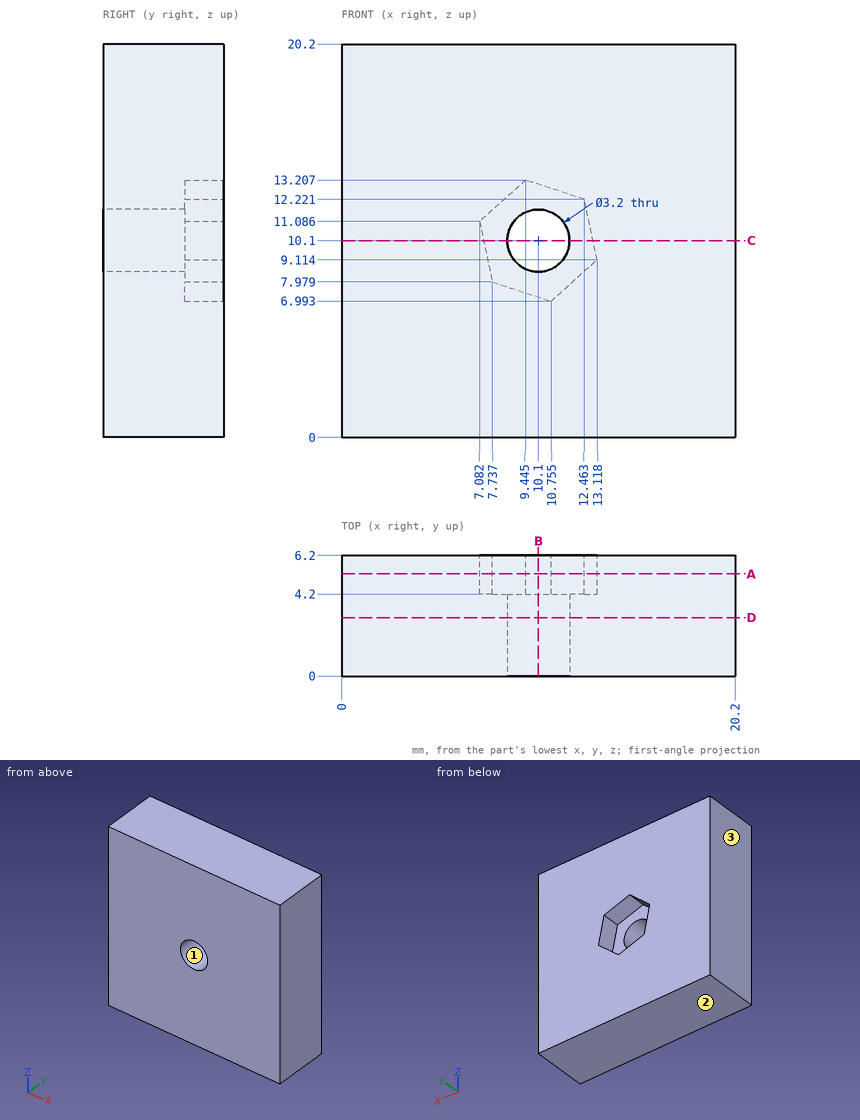
Here's the drawing with two shaded views (mm, measured from the low corner). I have some questions. Coordinates: 2 decimals unless noted, no trailing zeros. Write each loop counter-clockwise with the first axis right and the second up, starting at its lowest first coordinate (ties: lowest second). Pieces come first, ordered by that corner, then holes.
Item 1: I want a section at C-C on z = 10.1. Write out the boundary of the cut face in (x, y).
Item 2: I want a section at B-B on x = 10.1. Write out the boundary of the cut face in (y, z).
Item 3: If I drill on line 1 (Z direction, x = 10.1, y = 2.05); line 2 (Z direction, x = 11.5, y = 4.5) (1 decimal), over which ranges is the centre line in solid material (lowest first)?
Item 4: I want a section at D-D on y = 3. Write out the boundary of the cut face in (x, z), and give its area (3 significant figures).
Item 5: Will this pin go through, and if not, where does the flat tip stop? pin 1 (4 mm diameter, centred on x = 10.1, z = 10.1, fed in from +Y).
Item 6: If we mould it in two halves opening along Z, with no side actions, what happens to the marked faces 1, 2 and 3? For each: +Z half, -Z half, draft (parallel to the pull), parting line (faces both ways), or undercut.
Item 7: I want a section at A-A on y = 5.25. Write out the boundary of the cut face in (x, z) (1 decimal).
Findings below:
1. outline: (0, 0) - (8.5, 0) - (8.5, 4.2) - (7.29, 4.2) - (7.29, 6.2) - (0, 6.2) - close; (11.7, 0) - (20.2, 0) - (20.2, 6.2) - (12.91, 6.2) - (12.91, 4.2) - (11.7, 4.2) - close
2. outline: (0, 0) - (6.2, 0) - (6.2, 7.21) - (4.2, 7.21) - (4.2, 8.5) - (0, 8.5) - close; (0, 11.7) - (4.2, 11.7) - (4.2, 12.99) - (6.2, 12.99) - (6.2, 20.2) - (0, 20.2) - close
3. line 1: z = 0 to 8.5, 11.7 to 20.2
3. line 2: z = 0 to 7.7, 12.5 to 20.2
4. outline: (0, 0) - (20.2, 0) - (20.2, 20.2) - (0, 20.2) - close; hole circle Ø3.2 at (10.1, 10.1)
4. area: 400 mm2
5. pin 1: stops at y = 4.2
6. face 1: undercut
6. face 2: -Z half
6. face 3: draft
7. outline: (0, 0) - (20.2, 0) - (20.2, 20.2) - (0, 20.2) - close; hole (7.1, 11.1) - (7.7, 8) - (10.8, 7) - (13.1, 9.1) - (12.5, 12.2) - (9.4, 13.2) - close
